Input: dimensioned drawing with shaded views. Units: mm. Origin: part minimum x, y, z. Coordinates: 2 decimals unless noted, no trailing zeros. Order: outer loops, then holes, each group sorted by start corner. A loop starts at its lowest first (then second) coordinate and runs counter-clockwise, first axis right, second up.
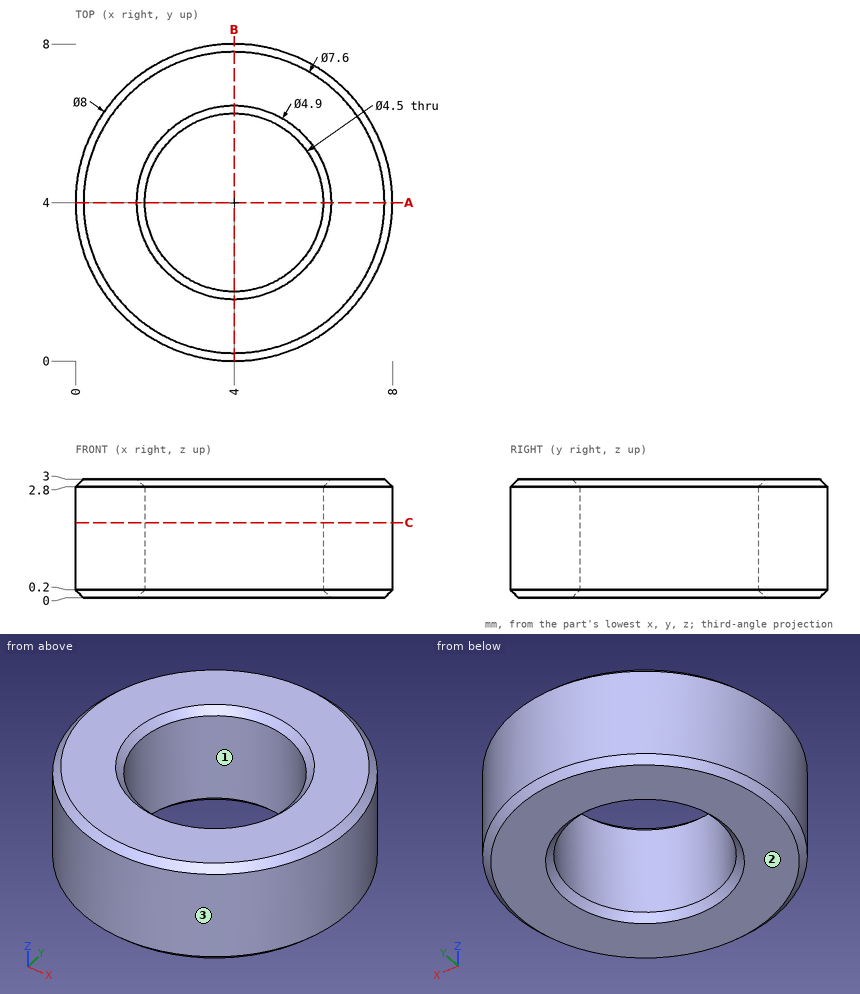
1. Section query C-C, the plane z = 1.9. Output: boundary loops of the cut face in (x, y).
2. Draft query along X for the marked faces 1, 2 and 3. Return one class per face: +X half, -X half, draft (parallel to the pull), parting line (faces both ways), or undercut.
3. Material intervals for line 1 along Y through (x, z) = (4, 1.65); line 2 along X through (y, z) = (4.5, 1.8); line 3 along X through (y, z) = (2, 2.35), sorted ascending.
4. Section query A-A, the plane y = 4. Output: boundary loops of the cut face in (x, z), plus the area to 3 significant figures.
Answer key:
1. outline: circle Ø8 at (4, 4); hole circle Ø4.5 at (4, 4)
2. face 1: undercut
2. face 2: draft
2. face 3: parting line
3. line 1: y = 0 to 1.75, 6.25 to 8
3. line 2: x = 0.03 to 1.81, 6.19 to 7.97
3. line 3: x = 0.54 to 2.97, 5.03 to 7.46
4. outline: (0, 0.2) - (0.2, 0) - (1.55, 0) - (1.75, 0.2) - (1.75, 2.8) - (1.55, 3) - (0.2, 3) - (0, 2.8) - close; (6.25, 0.2) - (6.45, 0) - (7.8, 0) - (8, 0.2) - (8, 2.8) - (7.8, 3) - (6.45, 3) - (6.25, 2.8) - close
4. area: 10.3 mm2
